from build123d import *

# Parameters (mm, degrees)
ESQUISSE1_W              = 85
ESQUISSE1_H              = 73
BOSS_EXTRU_2_DEPTH       = 2
ESQUISSE6_W              = 35
ESQUISSE6_H              = 73
BOSS_EXTRU_4_DEPTH       = 1
ESQUISSE8_W              = 35
ESQUISSE8_H              = 73
BOSS_EXTRU_6_DEPTH       = 1
ESQUISSE10_W             = 12
ESQUISSE10_H             = 11
ENL_V_MAT_EXTRU_1_DEPTH  = 1
ESQUISSE11_W             = 15
ESQUISSE11_H             = 13
ENL_V_MAT_EXTRU_2_DEPTH  = 1
ESQUISSE13_W             = 87
ESQUISSE13_H             = 35
BOSS_EXTRU_8_DEPTH       = 1
ESQUISSE14_W             = 12
ESQUISSE14_H             = 16
ENL_V_MAT_EXTRU_3_DEPTH  = 1
ESQUISSE18_W             = 12
ESQUISSE18_H             = 16
ENL_V_MAT_EXTRU_5_DEPTH  = 1
ESQUISSE20_W             = 12
ESQUISSE20_H             = 16
ENL_V_MAT_EXTRU_6_DEPTH  = 1
ESQUISSE21_W             = 12
ESQUISSE21_H             = 16
ENL_V_MAT_EXTRU_7_DEPTH  = 1
ESQUISSE25_W             = 87
ESQUISSE25_H             = 35
BOSS_EXTRU_11_DEPTH      = 1
ESQUISSE26_W             = 77
ESQUISSE26_H             = 22
ENL_V_MAT_EXTRU_13_DEPTH = 1
ESQUISSE23_R             = 3
ENL_V_MAT_EXTRU_14_DEPTH = 10
ESQUISSE22_R             = 3
ENL_V_MAT_EXTRU_15_DEPTH = 10
ESQUISSE24_R             = 3
ENL_V_MAT_EXTRU_18_DEPTH = 10
ESQUISSE27_W             = 10
ESQUISSE27_H             = 20
ENL_V_MAT_EXTRU_19_DEPTH = 1
ESQUISSE28_W             = 5
ESQUISSE28_H             = 6.5
ENL_V_MAT_EXTRU_20_DEPTH = 10


with BuildPart() as part:
    # Esquisse1 → Boss.-Extru.2 (new body)
    with BuildSketch(Plane.XY):
        with Locations((-89.704998798, 36.5)):
            Rectangle(ESQUISSE1_W, ESQUISSE1_H)
    extrude(amount=BOSS_EXTRU_2_DEPTH)

    # Esquisse6 → Boss.-Extru.4 (add)
    with BuildSketch(Plane(origin=(-47.204998798, 0, 0), x_dir=(0, 0, -1), z_dir=(1, 0, 0))):
        with Locations((-17.5, 36.5)):
            Rectangle(ESQUISSE6_W, ESQUISSE6_H)
    extrude(amount=BOSS_EXTRU_4_DEPTH)

    # Esquisse8 → Boss.-Extru.6 (add)
    with BuildSketch(Plane.ZY.offset(132.204998798)):
        with Locations((17.5, 36.5)):
            Rectangle(ESQUISSE8_W, ESQUISSE8_H)
    extrude(amount=BOSS_EXTRU_6_DEPTH)

    # Esquisse10 → Enlèv. mat.-Extru.1 (cut)
    with BuildSketch(Plane.ZY.offset(133.204998798)):
        with Locations((8, 59.5)):
            Rectangle(ESQUISSE10_W, ESQUISSE10_H)
    extrude(amount=-ENL_V_MAT_EXTRU_1_DEPTH, mode=Mode.SUBTRACT)

    # Esquisse11 → Enlèv. mat.-Extru.2 (cut)
    with BuildSketch(Plane.ZY.offset(133.204998798)):
        with Locations((9.5, 30.5)):
            Rectangle(ESQUISSE11_W, ESQUISSE11_H)
    extrude(amount=-ENL_V_MAT_EXTRU_2_DEPTH, mode=Mode.SUBTRACT)

    # Esquisse13 → Boss.-Extru.8 (add)
    with BuildSketch(Plane(origin=(0, 73, 0), x_dir=(1, 0, 0), z_dir=(0, 1, 0))):
        with Locations((-89.704998798, -17.5)):
            Rectangle(ESQUISSE13_W, ESQUISSE13_H)
    extrude(amount=BOSS_EXTRU_8_DEPTH)

    # Esquisse14 → Enlèv. mat.-Extru.3 (cut)
    with BuildSketch(Plane(origin=(0, 74, 0), x_dir=(1, 0, 0), z_dir=(0, 1, 0))):
        with Locations((-122.207040337, -26)):
            Rectangle(ESQUISSE14_W, ESQUISSE14_H)
    extrude(amount=-ENL_V_MAT_EXTRU_3_DEPTH, mode=Mode.SUBTRACT)

    # Esquisse18 → Enlèv. mat.-Extru.5 (cut)
    with BuildSketch(Plane(origin=(0, 74, 0), x_dir=(1, 0, 0), z_dir=(0, 1, 0))):
        with Locations((-108.207040337, -26)):
            Rectangle(ESQUISSE18_W, ESQUISSE18_H)
    extrude(amount=-ENL_V_MAT_EXTRU_5_DEPTH, mode=Mode.SUBTRACT)

    # Esquisse20 → Enlèv. mat.-Extru.6 (cut)
    with BuildSketch(Plane(origin=(0, 74, 0), x_dir=(1, 0, 0), z_dir=(0, 1, 0))):
        with Locations((-94.207040337, -26)):
            Rectangle(ESQUISSE20_W, ESQUISSE20_H)
    extrude(amount=-ENL_V_MAT_EXTRU_6_DEPTH, mode=Mode.SUBTRACT)

    # Esquisse21 → Enlèv. mat.-Extru.7 (cut)
    with BuildSketch(Plane(origin=(0, 74, 0), x_dir=(1, 0, 0), z_dir=(0, 1, 0))):
        with Locations((-80.207040337, -26)):
            Rectangle(ESQUISSE21_W, ESQUISSE21_H)
    extrude(amount=-ENL_V_MAT_EXTRU_7_DEPTH, mode=Mode.SUBTRACT)

    # Esquisse25 → Boss.-Extru.11 (add)
    with BuildSketch(Plane.XZ):
        with Locations((-89.704998798, 17.5)):
            Rectangle(ESQUISSE25_W, ESQUISSE25_H)
    extrude(amount=BOSS_EXTRU_11_DEPTH)

    # Esquisse26 → Enlèv. mat.-Extru.13 (cut)
    with BuildSketch(Plane.XZ.offset(1)):
        with Locations((-84.785991567, 11)):
            Rectangle(ESQUISSE26_W, ESQUISSE26_H)
    extrude(amount=-ENL_V_MAT_EXTRU_13_DEPTH, mode=Mode.SUBTRACT)

    # Esquisse23 → Enlèv. mat.-Extru.14 (cut)
    with BuildSketch(Plane.XY.offset(2)):
        with Locations((-128.228777758, 19.66052326)):
            Circle(ESQUISSE23_R)
    extrude(amount=-ENL_V_MAT_EXTRU_14_DEPTH, mode=Mode.SUBTRACT)

    # Esquisse22 → Enlèv. mat.-Extru.15 (cut)
    with BuildSketch(Plane.XY.offset(2)):
        with Locations((-128.334603856, 69.17039525)):
            Circle(ESQUISSE22_R)
    extrude(amount=-ENL_V_MAT_EXTRU_15_DEPTH, mode=Mode.SUBTRACT)

    # Esquisse24 → Enlèv. mat.-Extru.18 (cut)
    with BuildSketch(Plane.XY.offset(2)):
        with Locations((-70.21638406, 69.222983718)):
            Circle(ESQUISSE24_R)
    extrude(amount=-ENL_V_MAT_EXTRU_18_DEPTH, mode=Mode.SUBTRACT)

    # Esquisse27 → Enlèv. mat.-Extru.19 (cut)
    with BuildSketch(Plane.ZY.offset(133.204998798)):
        with Locations((25, 36.5)):
            Rectangle(ESQUISSE27_W, ESQUISSE27_H)
    extrude(amount=-ENL_V_MAT_EXTRU_19_DEPTH, mode=Mode.SUBTRACT)

    # Esquisse28 → Enlèv. mat.-Extru.20 (cut)
    with BuildSketch(Plane.ZY.offset(133.204998798)):
        with Locations((32.5, 36.5)):
            Rectangle(ESQUISSE28_W, ESQUISSE28_H)
    extrude(amount=-ENL_V_MAT_EXTRU_20_DEPTH, mode=Mode.SUBTRACT)


solid = part.part
Check sheet for the modelled part. Datum: model origin and axes. Units: mm. A direction names the side the tool comes from. Give positions to 0.01 mm unless a question says otherwise; leave off trailing zeros. Loops run counter-clockwise (first coordinate to the right, second up) from the corner with the lowest first, then second, coordinate; pieces in that order, holes last. Notation, with made-up numbers: M 82.5,10.5 L 141.5,10.5 A14 ccw 141.5,21.5 Z; hole C 74.25,78 d10. An arc over 180 degrees is marked long. Use a Markdown table: item, result. Add a question column.
Q1. Scan lines: line 1 along X through (y, z) = (21, 25.5) (3 decimals); line 2 along Y through (x, z) = (-116, 33.5); line 3 along Y through (x, z) = (-111.5, 15.5). Record each from-to range of solid material in increasing order. Write a range as [from, to].
Q2. Mould release check, pull along Y, two halves, no side actions. Record for faces 3 (the flat face through (-90, 74, 13)), 4 (the flat face through (-81, 73, 15)), 5 (the flat face through (-85, 0, 1)), 6 (the flat face through (-133.205, 37, 17.3)): pulls with the +Y half, pulls with the -Y half, needs draft (parallel to the pull), parting line crosses it, or undercut.
Q3. Sectioned sample at A-A, the plane y = 25. Record the cut outline in (x, z) (3 decimals), then the cut area to 3 significant figures.
Q4. Tool access check on faces 1 (the flat face through (-90, 0, 26)), 2 (the flat face through (-100, -1, 26)). Record the directions out of +Z, -Z, +X, -X, +Y, -Y that give a thin tool (end or side, any length) a straight path to the whole face; none if there is none.
Q5. Sectioned sample at D-D, the plane x = -93.5. Record the cut outline in (y, z), then the cut area to 3 significant figures.
Q6. Go/stop test with flat-tipped pins: pin 1 (16.5 mm diameter, centred on y = 28, z = 24.5, fed in from -X) (3 decimals); pin 2 (1.5 mm diameter, centred on x = -123.5, y = 47, fed in from +Z); pin 3 (4 mm diameter, centred on y = 33.5, z = 14, fed in from -X) (3 decimals). Record where each tip stops, or that it passes through.
Q7. Sectioned sample at C-C, the plane z = 6. Record the cut outline in (x, y) (3 decimals).
Q8. Sectioned sample at B-B, the plane x = -62. Record the cut outline in (y, z).
Verdict:
| question | item | result |
|---|---|---|
| 1 | line 1 | [-133.205, -132.205], [-47.205, -46.205] |
| 1 | line 2 | [-1, 0], [73, 74] |
| 1 | line 3 | [73, 74] |
| 2 | face 3 | pulls with the +Y half |
| 2 | face 4 | undercut |
| 2 | face 5 | pulls with the -Y half |
| 2 | face 6 | needs draft |
| 3 | outline | M -133.205,0 L -46.205,0 L -46.205,35 L -47.205,35 L -47.205,2 L -133.205,2 Z; M -133.205,17 L -132.205,17 L -132.205,35 L -133.205,35 Z |
| 3 | area | 225 mm^2 |
| 4 | face 1 | +Z |
| 4 | face 2 | +Z, -Z, +X, -X, -Y |
| 5 | outline | M -1,22 L 0,22 L 0,35 L -1,35 Z; M 0,0 L 74,0 L 74,18 L 73,18 L 73,2 L 0,2 Z; M 73,34 L 74,34 L 74,35 L 73,35 Z |
| 5 | area | 178 mm^2 |
| 6 | pin 1 | x = -133.205 |
| 6 | pin 2 | z = 2 |
| 6 | pin 3 | x = -47.205 |
| 7 | outline | M -133.205,-1 L -123.286,-1 L -123.286,0 L -132.205,0 L -132.205,24 L -133.205,24 Z; M -133.205,37 L -132.205,37 L -132.205,54 L -133.205,54 Z; M -133.205,65 L -132.205,65 L -132.205,73 L -47.205,73 L -47.205,0 L -46.286,0 L -46.286,-1 L -46.205,-1 L -46.205,74 L -133.205,74 Z |
| 8 | outline | M -1,22 L 0,22 L 0,35 L -1,35 Z; M 0,0 L 74,0 L 74,35 L 73,35 L 73,2 L 0,2 Z |
